Can you work these out from the drawing? Everything is in mm from the part's minimum corner. A direction names the side the tool comes from. Round coordinates to 2 decimals unless told otherwise and drop trailing zeros. Loops run counter-clockwise (first coordinate to the right, second up) from the corner with the lowest first, then second, coordinate; pieces in that order, holes last. Notation, with made-up numbers: M 17.25,11 L 67.25,11 A21 cw 67.25,42 Z; hole C 71.5,63 d6. An arc over 180 degrees is marked long. Return JSON: item names as keys, results as strings. Group by question number.
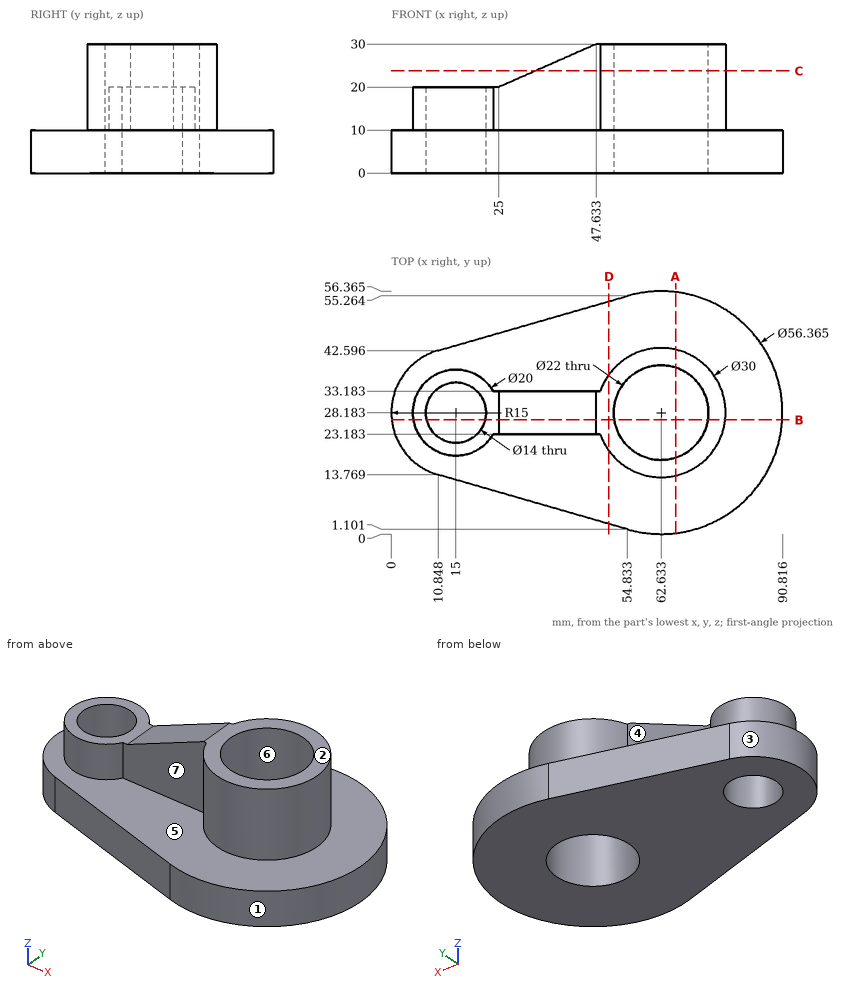
1. I need wall thicknesses on probe 1 along Z at (x, y) = (54, 41); probe 2 along Y at (x, z) = (55, 6.75) (1 decimal); probe 3 along Y at (x, z) = (59, 7.5) (1 decimal). Which ranges of each line are inside material? Lowest first, please.
2. We'd pull the mould along X, two halves only. Please class the marked faces 1, 2, 3 and 4: +X half, -X half, draft (parallel to the pull), parting line (faces both ways), or undercut.
3. I'm going to push flat-ended pins straight in: pin 1 Ø10 at (x, y) = (44, 44) entering from +Z; pin 2 Ø1.5 at (y, z) = (15, 21.5) entering from -X; pin 3 Ø6 at (x, z) = (36, 21) entering from -Y. Where does each tip first touch, or does it pass through?
4. If we section it at D-D, the plane x = 50.5: Please give me the cut outline in (y, z).
5. If we section it at A-A, the plane x = 66: Please give me the cut outline in (y, z) (1 decimal).
6. On a 3-axis mill with a long thin cutter (end or side, diameter ignored), from which of +Z, -Z, +X, -X, +Y, -Y can I reach the whole of each face in a straight line? I mean the marked faces 5, 6 and 7. Say none if no direction works.
7. If we section it at C-C, the plane z = 23.75: Please give me the cut outline in (x, y), then the cut area to 3 significant figures.
8. If we section it at B-B, the plane y = 26.5: Please give me the cut outline in (x, z) (1 decimal).
Geometry results:
{
 "1": {"probe 1": "0 to 10", "probe 2": "1.1 to 20.3, 36.1 to 55.3", "probe 3": "0.2 to 17.8, 38.6 to 56.1"},
 "2": {"face 1": "parting line", "face 2": "draft", "face 3": "-X half", "face 4": "undercut"},
 "3": {"pin 1": "z = 10", "pin 2": "x = 54.24", "pin 3": "y = 23.18"},
 "4": {"outline": "M 2.35,0 L 54.02,0 L 54.02,10 L 37,10 L 37,30 L 19.36,30 L 19.36,10 L 2.35,10 Z"},
 "5": {"outline": "M 0.2,0 L 17.7,0 L 17.7,30 L 13.6,30 L 13.6,10 L 0.2,10 Z; M 38.7,0 L 56.2,0 L 56.2,10 L 42.8,10 L 42.8,30 L 38.7,30 Z"},
 "6": {"face 5": "+Z", "face 6": "+Z, -Z", "face 7": "+Z, -Y"},
 "7": {"outline": "M 33.49,23.18 L 48.49,23.18 A15 ccw long 48.49,33.18 L 33.49,33.18 Z; hole C 62.63,28.18 d22", "area": "471 mm^2"},
 "8": {"outline": "M 0.1,0 L 8.2,0 L 8.2,20 L 5.1,20 L 5.1,10 L 0.1,10 Z; M 21.8,0 L 51.8,0 L 51.8,30 L 47.6,30 L 25,20 L 21.8,20 Z; M 73.5,0 L 90.8,0 L 90.8,10 L 77.5,10 L 77.5,30 L 73.5,30 Z"}
}
